Check sheet for the modelled part. Datum: model origin and axes. Units: mm. Give positions to 0.01 mm unless a question says otherwise; leave off trailing zeros. Loops run counter-clockwise (first coordinate to the right, second up) from the corner with the lowest first, then second, coordinate; pieces in that order, holes last.
```python
from build123d import *

# Parameters (mm, degrees)
BOSS_EXTRUDE2_DEPTH   = 5
F_6_CLEARANCE_HOLE1_D = 3.7973


with BuildPart() as part:
    # Sketch2 → Boss-Extrude2 (new body)
    with BuildSketch(Plane(origin=(0, 0, 0), x_dir=(1, 0, 0), z_dir=(0, 1, 0))):
        with BuildLine():
            ThreePointArc((-1.921673483, -7.798539123), (3.967844549, -11.837003018), (9.548776015, -7.381801872))
            Line((9.548776015, -7.381801872), (10.998470019, -1.926053578))
            ThreePointArc((10.998470019, -1.926053578), (11.24988985, -0.04064778), (11.018921171, 1.84737246))
            Line((11.018921171, 1.84737246), (9.565136937, 7.567628243))
            ThreePointArc((9.565136937, 7.567628243), (3.75, 12.089730275), (-2.065136937, 7.567628243))
            Line((-2.065136937, 7.567628243), (-3.518921171, 1.84737246))
            ThreePointArc((-3.518921171, 1.84737246), (-3.749830525, -0.050419155), (-3.493426606, -1.944934706))
            Line((-3.493426606, -1.944934706), (-1.921673483, -7.798539123))
        make_face()
    extrude(amount=BOSS_EXTRUDE2_DEPTH)

    # #6 Clearance Hole1 (through all)
    with Locations(Plane(origin=(0, 5, 0), x_dir=(1, 0, 0), z_dir=(0, 1, 0))):
        with Locations((3.75, 6.089730275), (3.75, -5.840959009)):
            Hole(F_6_CLEARANCE_HOLE1_D / 2)


solid = part.part
```
(1) Section check D-D on x = 0.75. Record the boundary of the cut face in (y, z), plus the area to 3 significant figures.
(2) Section check C-C on y = 2.2. Record the boundary of the cut face in (x, z), plus the area to 3 significant figures.
(3) Material ranges on line 1 (Z direction, x = 3.75, y = 3.4); line 2 (Z direction, x = 3.5, y = 3); line 3 (X direction, y = 0.3, z = 4.5), recorded low to high.
(4) Release check for a two-part mould opening along Z. For faces 1 (the face through (-2.78, 2.46, -4.75)), 2 (the face through (3.86, 2.46, 11.84)), 3 (the face through (2.874, 2.465, 7.525)) record: pulls with the +Z half, pulls with the -Z half, needs draft (parallel to the pull), parting line crosses it, or undercut.
(5) Section check A-A on x = 3.75. Record the boundary of the cut face in (y, z), plus the area to 3 significant figures.
(6) Section check B-B on z = 4.5. Record the boundary of the cut face in (x, y), plus the area to 3 significant figures.
Computed values:
1. outline: (0, -11.29) - (5, -11.29) - (5, 11.04) - (0, 11.04) - close
1. area: 112 mm2
2. outline: (-3.52, -1.85) - (-2.07, -7.57) arc R6 ccw to (9.57, -7.57) - (11.02, -1.85) arc R7.5 ccw to (11, 1.93) - (9.55, 7.38) arc R6 ccw to (-1.92, 7.8) - (-3.49, 1.94) arc R7.5 ccw to start; hole circle Ø3.8 at (3.75, -6.09); hole circle Ø3.8 at (3.75, 5.84)
2. area: 257 mm2
3. line 1: z = -12.09 to -7.99, -4.19 to 3.94, 7.74 to 11.84
3. line 2: z = -12.08 to -7.97, -4.21 to 3.96, 7.72 to 11.84
3. line 3: x = -2.81 to 2.41, 5.09 to 10.31
4. face 1: pulls with the -Z half
4. face 2: pulls with the +Z half
4. face 3: undercut
5. outline: (0, -12.09) - (5, -12.09) - (5, -7.99) - (0, -7.99) - close; (0, -4.19) - (5, -4.19) - (5, 3.94) - (0, 3.94) - close; (0, 7.74) - (5, 7.74) - (5, 11.84) - (0, 11.84) - close
5. area: 81.7 mm2
6. outline: (-2.81, 0) - (2.41, 0) - (2.41, 5) - (-2.81, 5) - close; (5.09, 0) - (10.31, 0) - (10.31, 5) - (5.09, 5) - close
6. area: 52.2 mm2
